```python
from build123d import *

# Parameters (mm, degrees)
SKETCH2_R           = 7
SKETCH2_R_2         = 5
BOSS_EXTRUDE1_DEPTH = 2
SKETCH2_3_R         = 5
SKETCH2_3_R_2       = 4.5
BOSS_EXTRUDE2_DEPTH = 1.5
SKETCH2_4_R         = 4.5
SKETCH2_4_R_2       = 2.5
BOSS_EXTRUDE3_DEPTH = 2


with BuildPart() as part:
    # Sketch2 → Boss-Extrude1 (new, symmetric)
    with BuildSketch(Plane(origin=(0, 0, 0), x_dir=(0, 0, -1), z_dir=(1, 0, 0))):
        Circle(SKETCH2_R)
        Circle(SKETCH2_R_2, mode=Mode.SUBTRACT)
    extrude(amount=BOSS_EXTRUDE1_DEPTH, both=True)

    # Sketch2<3> → Boss-Extrude2 (add, symmetric)
    with BuildSketch(Plane(origin=(0, 0, 0), x_dir=(0, 0, -1), z_dir=(1, 0, 0))):
        Circle(SKETCH2_3_R)
        Circle(SKETCH2_3_R_2, mode=Mode.SUBTRACT)
    extrude(amount=BOSS_EXTRUDE2_DEPTH, both=True)

    # Sketch2<4> → Boss-Extrude3 (add, symmetric)
    with BuildSketch(Plane(origin=(0, 0, 0), x_dir=(0, 0, -1), z_dir=(1, 0, 0))):
        Circle(SKETCH2_4_R)
        Circle(SKETCH2_4_R_2, mode=Mode.SUBTRACT)
    extrude(amount=BOSS_EXTRUDE3_DEPTH, both=True)


solid = part.part
```
Verification items for the finished model (mm, model axes). A direction names the side the tool comes from. Give positions to 0.01 mm unless a question says otherwise; leave off trailing zeros. Order: outer loops, then holes, each group sorted by start corner. A loop starts at its lowest first (then second) coordinate and runs counter-clockwise, first axis right, second up. Notation, with made-up numbers: (45.5, 7) -> (86.5, 7) arc R24 cw to (86.5, 33) -> close; hole circle Ø3 at (77, 48). An arc over 180 degrees is marked (long way). One line per item, written item: value.
(1) Gauge pin test, flat ends, axial feed: pin 1 (1.5 mm diameter, centred on x = 1.5, z = -2.5, fed in from -Y); pin 2 (2 mm diameter, centred on x = 0.5, y = 2.5, fed in from -Z); pin 3 (1 mm diameter, centred on x = -1, z = -5, fed in from +Y). Record the tip position at first contact, or that the pin passes through.
Final values:
pin 1: y = -6.78
pin 2: z = -6.84
pin 3: y = 5.36
(2) Draft check along Z on faces 1 (the face through (0.028, -2.681, -6.466)), 2 (the face through (-0.03, -2.44, 0.54)), 3 (the face through (-2, 5, 2)). Enter one of: pulls with the +Z half, pulls with the -Z half, needs draft (parallel to the pull), parting line crosses it, or undercut.
Final values:
face 1: parting line crosses it
face 2: undercut
face 3: needs draft
(3) Sectioned sample at D-D on z = -3. Record the cut outline in (x, y), then the cut area to 3 significant figures.
Final values:
outline: (-2, -6.32) -> (2, -6.32) -> (2, -4) -> (1.5, -4) -> (1.5, -3.35) -> (2, -3.35) -> (2, 3.35) -> (1.5, 3.35) -> (1.5, 4) -> (2, 4) -> (2, 6.32) -> (-2, 6.32) -> (-2, 4) -> (-1.5, 4) -> (-1.5, 3.35) -> (-2, 3.35) -> (-2, -3.35) -> (-1.5, -3.35) -> (-1.5, -4) -> (-2, -4) -> close
area: 49.3 mm^2
(4) Scan lines: line 1 along Y through (x, z) = (-1.65, 0); line 2 along Z through (x, y) = (1.85, 1); line 3 along Y through (x, z) = (-0.6, 0). Record each from-to range of solid material in increasing order. Write a range as [from, to].
Final values:
line 1: [-7, -5], [-4.5, -2.5], [2.5, 4.5], [5, 7]
line 2: [-6.93, -4.9], [-4.39, -2.29], [2.29, 4.39], [4.9, 6.93]
line 3: [-7, -2.5], [2.5, 7]
(5) Sectioned sample at C-C on x = 0.2. Record the cut outline in (y, z), then the cut area to 3 significant figures.
Final values:
outline: circle Ø14 at (0, 0); hole circle Ø5 at (0, 0)
area: 134 mm^2
(6) Sectioned sample at A-A on z = 0. Record the cut outline in (x, y).
Final values:
outline: (-2, -7) -> (2, -7) -> (2, -5) -> (1.5, -5) -> (1.5, -4.5) -> (2, -4.5) -> (2, -2.5) -> (-2, -2.5) -> (-2, -4.5) -> (-1.5, -4.5) -> (-1.5, -5) -> (-2, -5) -> close; (-2, 2.5) -> (2, 2.5) -> (2, 4.5) -> (1.5, 4.5) -> (1.5, 5) -> (2, 5) -> (2, 7) -> (-2, 7) -> (-2, 5) -> (-1.5, 5) -> (-1.5, 4.5) -> (-2, 4.5) -> close
(7) Tool access check on faces 4 (the face through (1.75, -4.88, 1.08)), 5 (the face through (-1.75, 4.46, 0.59)), 6 (the face through (2, 5, 2)). Record the directions out of +Z, -Z, +X, -X, +Y, -Y that give a thin tool (end or side, any length) a straight path to the whole face; none if there is none.
Final values:
face 4: +X
face 5: -X
face 6: +Z, -Z, +X, +Y, -Y
